Autodesk Inventor part; units mm, degrees
ref_plane "YZ Plane" through (0, 0, 0) normal (1, 0, 0) x (0, 1, 0)
ref_plane "XZ Plane" through (0, 0, 0) normal (0, 1, 0) x (-1, 0, 0)
ref_plane "XY Plane" through (0, 0, 0) normal (0, 0, 1) x (1, 0, 0)
sketch "Sketch1" plane through (0, 0, 0) normal (1, 0, 0) x (0, 1, 0)
  line L0 (-5, 6) -> (5, 6)
  line L1 (5, 6) -> (5, -6)
  line L2 (5, -6) -> (-5, -6)
  line L3 (-5, -6) -> (-5, 6)
  line L4 (-5, 6) -> (5, -6) construction
  line L5 (5, 6) -> (-5, -6) construction
  point P0 (0, 0)
  dimension "d0" = 10
  dimension "d1" = 12
extrude "Extrusion1" add sketch "Sketch1" along normal blind 29
sketch "Sketch2" plane through (0, 0, 0) normal (-1, 0, 0) x (0, 0, 1)
  circle A0 centre (0, 0) radius 2
  dimension "d4" = 4
extrude "Extrusion2" add sketch "Sketch2" along normal blind 1
sketch "Sketch3" plane through (-1, 0, 0) normal (-1, 0, 0) x (0, 0, 1)
  circle A0 centre (0, 0) radius 1.5
  dimension "d7" = 3
extrude "Extrusion3" add sketch "Sketch3" along normal blind 9
properties part number "Micro Gear motor" material "Copper, Alloy"
Read the model definition and answer for the solid it produces. Units are mm, in the model's axes. A direction names the side the tool comes from. Give positions to 0.01 mm unless a question says otherwise; leave off trailing zeros. Write each loop counter-clockwise with the first axis right and the second up, starting at its lowest first coordinate (ties: lowest second). Pieces come first, ordered by that corner, then holes. Notation, with made-up numbers: (27.25, 28) -> (35.25, 28) arc R8 ccw to (35.25, 39) -> close; hole circle Ø8 at (29.25, 70). An arc over 180 degrees is marked (long way). Answer in a Markdown table with one row per item.
1) A tool of negligible diameter and unlimited length cuts with its end or side. For faces 1 (the cylindrical face through (-0.493, 1.952, -0.434)), 2 (the flat face through (14, 0, 6)), from which of +Z, -Z, +X, -X, +Y, -Y can it reach the whole face along a straight path? Write none if from no direction.
Results list:
| item | result |
|---|---|
| face 1 | -X |
| face 2 | +Z, +X, -X, +Y, -Y |
2) Section A-A on y = 0 is taken. Give the vertices of the cut face in (x, z), plus the area to 3 significant figures.
Results list:
| item | result |
|---|---|
| outline | (-10, -1.5) -> (-1, -1.5) -> (-1, -2) -> (0, -2) -> (0, -6) -> (29, -6) -> (29, 6) -> (0, 6) -> (0, 2) -> (-1, 2) -> (-1, 1.5) -> (-10, 1.5) -> close |
| area | 379 mm^2 |
3) Section B-B on z = 0 is taken. Give the vertices of the cut face in (x, y), plus the area to 3 significant figures.
Results list:
| item | result |
|---|---|
| outline | (-10, -1.5) -> (-1, -1.5) -> (-1, -2) -> (0, -2) -> (0, -5) -> (29, -5) -> (29, 5) -> (0, 5) -> (0, 2) -> (-1, 2) -> (-1, 1.5) -> (-10, 1.5) -> close |
| area | 321 mm^2 |
4) Straight lines are drawn through the part: line 1 (X direction, y = 2.25, z = 3.5); line 2 (Y direction, x = -3.5, z = -1); line 3 (Z direction, x = -6, y = -0.5). For each, find the intervals that lie inside material, in ascending order. Write a range as [from, to].
Results list:
| item | result |
|---|---|
| line 1 | [0, 29] |
| line 2 | [-1.12, 1.12] |
| line 3 | [-1.41, 1.41] |
5) Section D-D on y = 3.5 is taken. Give the vertices of the cut face in (x, z), plus the area to 3 significant figures.
Results list:
| item | result |
|---|---|
| outline | (0, -6) -> (29, -6) -> (29, 6) -> (0, 6) -> close |
| area | 348 mm^2 |
6) Section C-C on x = -4 is taken. Give the vertices of the cut face in (y, z).
Results list:
| item | result |
|---|---|
| outline | circle Ø3 at (0, 0) |
